Work out the finished part from the listing and answer in its coordinate system (mm). A direction names the side the tool comes from. Round coordinates to 2 decimals unless told otherwise and drop trailing zeros. Loops run counter-clockwise (first coordinate to the right, second up) from the corner with the lowest first, then second, coordinate; pieces in that order, holes last. Notation, with made-up numbers: M 64.25,89.25 L 103.25,89.25 A8 ccw 103.25,95.25 Z; hole C -9,78 d4. An arc over 180 degrees is marked long. One line per item, written item: value.
```python
from build123d import *

# Parameters (mm, degrees)
F0_W          = 5
F0_H          = 60
F1_DEPTH      = 25
F1_DEPTH_BACK = 25
F2_W          = 50
F2_H          = 10
F3_DEPTH      = 40
F5_DEPTH      = 25
F6_R          = 2
F8_D          = 3.3
F10_DEPTH     = 60


with BuildPart() as f1:
    # F0 (on Right) → F1 (new body, two sides)
    with BuildSketch(Plane.YZ) as f1_sk:
        Rectangle(F0_W, F0_H)
    extrude(amount=F1_DEPTH)
    extrude(f1_sk.sketch, amount=-F1_DEPTH_BACK)

    # F2 (on Front) → F3 (join)
    with BuildSketch(Plane.XZ):
        with Locations((0, -25)):
            Rectangle(F2_W, F2_H)
    extrude(amount=F3_DEPTH)

    # F4 (on face) → F5 (cut)
    with BuildSketch(Plane.XY.offset(-20)):
        with BuildLine():
            ThreePointArc((6.25, -20), (0, -26.25), (-6.25, -20))
            Line((-6.25, -20), (-6.25, -40))
            Line((-6.25, -40), (6.25, -40))
            Line((6.25, -40), (6.25, -20))
        make_face()
        with BuildLine():
            ThreePointArc((6.25, -20), (0, -13.75), (-6.25, -20))
            ThreePointArc((-6.25, -20), (0, -26.25), (6.25, -20))
        make_face()
    extrude(amount=-F5_DEPTH, mode=Mode.SUBTRACT)

    # F6
    f6_edges = [f1.edges().sort_by_distance(p)[0] for p in [
        (-25, -21.25, -20),
        (-25, -2.5, 5),
        (25, -21.25, -20),
        (25, -2.5, 5),
        (-15.625, -40, -20),
        (15.625, -40, -20),
        (-15.625, -40, -30),
        (-25, -18.75, -30),
        (25, -18.75, -30),
        (15.625, -40, -30),
        (25, -40, -25),
        (-25, -40, -25),
        (0, -2.5, 30),
        (0, -2.5, -20),
    ]]
    fillet(f6_edges, radius=F6_R)

    # F8 (through all)
    with Locations(Plane.XY.offset(-20)):
        with Locations((-11, -19.460708499), (11, -19.460708499), (11, -34.460708499), (-11, -34.460708499)):
            Hole(F8_D / 2)

    # F9 (on face) → F10 (join)
    with BuildSketch(Plane.XY.offset(30)):
        Polygon((-25, 7.5), (-25, -0.5), (25, -0.5), (25, 7.5), (17.5, 7.5), (20, 2.5), (-20, 2.5), (-17.5, 7.5), align=None)
    extrude(amount=-F10_DEPTH)


solid = f1.part
```
1) Find the intervals of material crossed by probe 1 along Y at (x, z) = (11, -25); probe 2 along Y at (x, z) = (9.5, -11); probe 3 along Z at (x, y) = (-10.5, -24.5), in increasing order. Write a range as from..to.
Check values:
probe 1: -40..-36.11, -32.81..-21.11, -17.81..2.5
probe 2: -2.5..2.5
probe 3: -30..-20
2) For faces 1 (the face through (-24.43, -21.48, -20.6)), 2 (the face through (18.732, 5.035, 0.42)), 3 (the face through (-6.25, -30, -25)), determine the directions among +Z, -Z, +X, -X, +Y, -Y from which every point of the face is accessible in a straight line to the end or side of a thin tool.
Check values:
face 1: +Z, -X, -Y
face 2: +Z, -Z
face 3: +Z, -Z, -Y
3) Each of these flat-tipped pins is pushed along its axis until it touches: pin 1 (4.5 mm diameter, centred on x = 11, y = -19.46, fed in from -Z); pin 2 (2 mm diameter, centred on x = 23.5, z = -29, fed in from -Y); pin 3 (3 mm diameter, centred on x = -13, z = 7, fed in from -Y); pin 4 (20 mm diameter, centred on x = -6.5, z = 5, fed in from +Y). Where does it stop, or does it pass through?
Check values:
pin 1: z = -30
pin 2: y = -40
pin 3: y = -2.5
pin 4: y = 2.5
4) Find section B-B (x = 11). Give the vertices of the cut face in (y, z).
Check values:
outline: M -40,-28 A2 ccw -38,-30 L -36.11,-30 L -36.11,-20 L -38,-20 A2 ccw -40,-22 Z; M -32.81,-30 L -21.11,-30 L -21.11,-20 L -32.81,-20 Z; M -17.81,-30 L 2.5,-30 L 2.5,30 L -0.5,30 A2 ccw -2.5,28 L -2.5,-18 A2 cw -4.5,-20 L -17.81,-20 Z
5) Find section C-C (z = 4). Give the vertices of the cut face in (x, y), then the cut area to 3 significant figures.
Check values:
outline: M -25,-0.5 A2 ccw -23,-2.5 L 23,-2.5 A2 ccw 25,-0.5 L 25,7.5 L 17.5,7.5 L 20,2.5 L -20,2.5 L -17.5,7.5 L -25,7.5 Z
area: 311 mm2
6) Find section A-A (y = 4.5). Give the vertices of the cut face in (x, z), then the cut area to 3 significant figures.
Check values:
outline: M -25,-30 L -19,-30 L -19,30 L -25,30 Z; M 19,-30 L 25,-30 L 25,30 L 19,30 Z
area: 720 mm2
7) The mould has two halves that part along Y. Classify faces 4 (the face through (24.4, -19.51, -29.43)), 5 (the face through (10.239, -35.925, -25.07)), 6 (the face through (15, -40, -25)): +Y half, -Y half, draft (parallel to the pull), parting line (faces both ways), or undercut.
Check values:
face 4: draft
face 5: undercut
face 6: -Y half
8) Find section D-D (y = -24). Give the vertices of the cut face in (x, z), then the cut area to 3 significant figures.
Check values:
outline: M -25,-28 A2 ccw -23,-30 L -6.25,-30 L -6.25,-20 L -23,-20 A2 ccw -25,-22 Z; M 6.25,-30 L 23,-30 A2 ccw 25,-28 L 25,-22 A2 ccw 23,-20 L 6.25,-20 Z
area: 372 mm2
